from build123d import *

# Parameters (mm, degrees)
F0_W      = 76.2
F0_H      = 76.2
F1_DEPTH  = 76.2
F2_W      = 25.4
F2_H      = 25.4
F3_DEPTH  = 12.7
F4_R      = 12.7
F5_DEPTH  = 12.7
F8_D      = 25.4
F10_DEPTH = 12.7


with BuildPart() as f1:
    # F0 (on Front) → F1 (new body)
    with BuildSketch(Plane.XZ):
        with Locations((-38.1, 38.1)):
            Rectangle(F0_W, F0_H)
    extrude(amount=F1_DEPTH)

    # F2 (on face) → F3 (join)
    with BuildSketch(Plane.XZ.offset(76.2)):
        with Locations((-38.1, 38.1)):
            Rectangle(F2_W, F2_H)
    extrude(amount=F3_DEPTH)

    # F4 (on face) → F5 (join)
    with BuildSketch(Plane.YZ):
        with Locations((-38.1, 38.1)):
            Circle(F4_R)
    extrude(amount=F5_DEPTH)

    # F8 (through all)
    with Locations(Plane.XY.offset(76.2)):
        with Locations((-38.1, -38.1)):
            Hole(F8_D / 2)

    # F9 (on face) → F10 (join)
    with BuildSketch(Plane(origin=(-76.2, 0, 0), x_dir=(0, -1, 0), z_dir=(-1, 0, 0))):
        Polygon((38.1, 50.8), (25.593038, 28.692628), (50.98917, 29.135919), align=None)
    extrude(amount=F10_DEPTH)


solid = f1.part
The model under review builds one solid part; all positions refer to its coordinate system, in mm. A direction names the side the tool comes from. Coordinates: 2 decimals unless noted, no trailing zeros. Write each loop counter-clockwise with the first axis right and the second up, starting at its lowest first coordinate (ties: lowest second). Pieces come first, ordered by that corner, then holes. Notation, with made-up numbers: (-1.5, -0.75) -> (16.5, -0.75) arc R24 cw to (16.5, 34.25) -> close; hole circle Ø3 at (-1, 34.25). An arc over 180 degrees is marked (long way). Answer in a Markdown table with one row per item.
1. We need section C-C, the plane x = -31. State the section outline as (y, z) points, and give its area (3 significant figures).
Answers below:
| item | result |
|---|---|
| outline | (-88.9, 25.4) -> (-76.2, 25.4) -> (-76.2, 0) -> (-48.63, 0) -> (-48.63, 76.2) -> (-76.2, 76.2) -> (-76.2, 50.8) -> (-88.9, 50.8) -> close; (-27.57, 0) -> (0, 0) -> (0, 76.2) -> (-27.57, 76.2) -> close |
| area | 4,520 mm^2 |
2. For faces 1 (the flat face through (-38, -82, 50.8)), 2 (the flat face through (-82.461, -44.635, 39.816)), 3 (the flat face through (-25.4, -82, 38)), 4 (the flat face through (-50.8, -82, 38)), 5 (the flat face through (-38, -82, 25.4)), list the 3-axis set-ups (+Z, -Z, +X, -X, +Y, -Y) from which the entire face can be reached by the end or side of a thin tool; tool diameter is ignored.
Answers below:
| item | result |
|---|---|
| face 1 | +Z, +X, -X, -Y |
| face 2 | +Z, -X, -Y |
| face 3 | +Z, -Z, +X, -Y |
| face 4 | +Z, -Z, -X, -Y |
| face 5 | -Z, +X, -X, -Y |
3. We need section A-A, the plane z = 45.5. State the section outline as (x, y) points.
Answers below:
| item | result |
|---|---|
| outline | (-88.9, -41.25) -> (-76.2, -41.25) -> (-76.2, -76.2) -> (-50.8, -76.2) -> (-50.8, -88.9) -> (-25.4, -88.9) -> (-25.4, -76.2) -> (0, -76.2) -> (0, -48.42) -> (12.7, -48.42) -> (12.7, -27.78) -> (0, -27.78) -> (0, 0) -> (-76.2, 0) -> (-76.2, -35.1) -> (-88.9, -35.1) -> close; hole circle Ø25.4 at (-38.1, -38.1) |
4. Clearance check with flat-ended pins moving along their axes: pin 1 Ø3 at (y, z) = (-76.5, 34) entering from +X; pin 2 Ø10 at (x, y) = (-32, -83) entering from +Z; pin 3 Ø4 at (y, z) = (-83, 43) entering from -X. State where each tip first meets the part, or that it passes through.
Answers below:
| item | result |
|---|---|
| pin 1 | stops at x = 0 |
| pin 2 | stops at z = 50.8 |
| pin 3 | stops at x = -50.8 |
5. We need section B-B, the plane y = -42. State the section outline as (x, z) points.
Answers below:
| item | result |
|---|---|
| outline | (-88.9, 28.98) -> (-76.2, 28.98) -> (-76.2, 0) -> (-50.19, 0) -> (-50.19, 76.2) -> (-76.2, 76.2) -> (-76.2, 44.24) -> (-88.9, 44.24) -> close; (-26.01, 0) -> (0, 0) -> (0, 26.01) -> (12.7, 26.01) -> (12.7, 50.19) -> (0, 50.19) -> (0, 76.2) -> (-26.01, 76.2) -> close |
6. Wall thickness on probe 1 along Y at (x, z) = (-38, 41); probe 2 along Y at (x, z) = (-38.1, 25); probe 3 along X at (y, z) = (-38.5, 39): over which ranges is each line inside the solid? List them lowest first. Write a range as [from, to].
Answers below:
| item | result |
|---|---|
| probe 1 | y = [-88.9, -50.8], [-25.4, 0] |
| probe 2 | y = [-76.2, -50.8], [-25.4, 0] |
| probe 3 | x = [-88.9, -50.79], [-25.41, 12.7] |
7. We need section D-D, the plane y = -83. State the section outline as (x, z) points, and give its area (3 significant figures).
Answers below:
| item | result |
|---|---|
| outline | (-50.8, 25.4) -> (-25.4, 25.4) -> (-25.4, 50.8) -> (-50.8, 50.8) -> close |
| area | 645 mm^2 |
